Autodesk Inventor part; units mm, degrees
ref_plane "YZ Plane" through (0, 0, 0) normal (1, 0, 0) x (0, 1, 0)
ref_plane "XZ Plane" through (0, 0, 0) normal (0, 1, 0) x (-1, 0, 0)
ref_plane "XY Plane" through (0, 0, 0) normal (0, 0, 1) x (1, 0, 0)
sketch "スケッチ1" plane through (0, 0, 0) normal (0, 0, 1) x (1, 0, 0)
  line L0 (0, 0) -> (62, 0) construction
  line L1 (62, 0) -> (62, -62) construction
  line L2 (62, -62) -> (0, -62) construction
  line L3 (0, -62) -> (0, 0) construction
  line L4 (20.6, -15.3248) -> (42.6, -15.3248)
  line L5 (42.6, -15.3248) -> (42.6, -53.3248)
  line L6 (42.6, -53.3248) -> (20.6, -53.3248)
  line L7 (20.6, -53.3248) -> (20.6, -15.3248)
  circle A0 centre (26.9, -25.5248) radius 4.25
  circle A1 centre (36.3, -25.5248) radius 4.25
  dimension "d1" = 22
  dimension "d2" = 38
  dimension "d3" = 62
  dimension "d12" = 15.3248
  dimension "d16" = 20.6
  dimension "d17" = 8.5
  dimension "d18" = 8.5
  dimension "d19" = 6.3
  dimension "d25" = 10.2
  dimension "d31" = 6.3
extrude "押し出し1" add sketch "スケッチ1" along normal blind 5
sketch "スケッチ2" plane through (0, 0, 0) normal (0, 0, -1) x (-1, 0, 0)
  circle A0 centre (-36.3, -25.5248) radius 4.25
  circle A1 centre (-26.9, -25.5248) radius 4.25
  point P0 (0, 0)
extrude "押し出し2" add sketch "スケッチ2" against normal blind 12.7
equation "\"d17\" = d18"
equation "\"d31\" = d19"
properties part number "sidewindermicro2"
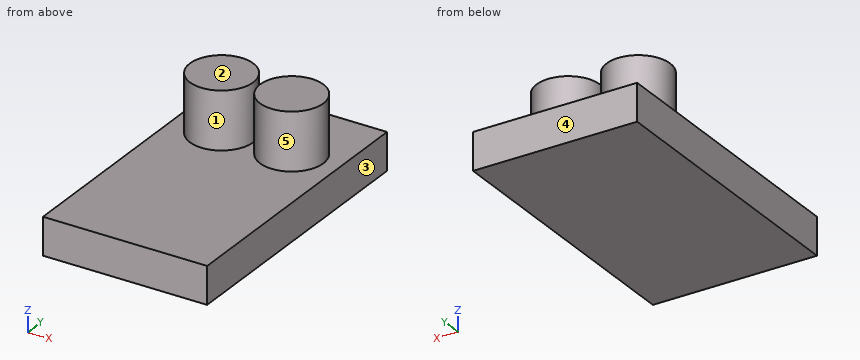
Geometry check sheet. Reference: the model listing, model coordinates, mm. Face numbers are marked on the shaded views. A direction names the side the tool comes from. Round coordinates to 2 decimals unless told otherwise and drop trailing zeros. Loops run counter-clockwise (first coordinate to the right, second up) from the corner with the lowest first, then second, coordinate; pieces in that order, holes last. Notation, with made-up numbers: M 26,25.25 L 47,25.25 A35 ccw 47,57.25 Z; hole C 35,-14.75 d7. An arc over 180 degrees is marked long. Return JSON: item names as keys, results as strings. Group by question number.
(1) Section check A-A, the plane x = 26.9. Enter the section's corners in (y, z), and give its area (3 significant figures).
(2) Go/stop test with flat-tipped pins: pin 1 (3 mm diameter, centred on x = 28.5, y = -21, fed in from -Z); pin 2 (1 mm diameter, centred on y = -22, z = 6, fed in from +X); pin 3 (5 mm diameter, centred on x = 33.5, z = 8.5, fed in from +Y). Record where each tip stops, or that it passes through.
(3) Scan lines: line 1 along Z through (x, y) = (24.5, -35.5); line 2 along X through (y, z) = (-22, 11.25); line 3 along Y through (x, z) = (35.75, 9). Record each from-to range of solid material in increasing order. Write a range as [from, to].
(4) Mould release check, pull along X, two halves, no side actions. Record for the marked faces 1, 2 and 3: pulls with the +X half, pulls with the -X half, needs draft (parallel to the pull), parting line crosses it, or undercut.
(5) Set-up check for the marked faces 4 and 5: record each of +Z, -Z, +X, -X, +Y, -Y from which the full face is reachable in a straight line by a thin tool's end or side.
(6) Section check C-C, the plane z = 8. Enter the section's corners in (x, y).
(7) Section check D-D, the plane x = 22.25. Enter the section's corners in (y, z), and give its area (3 significant figures).
(8) Section check B-B, the plane y = -22. Enter the section's corners in (x, z).
Data:
{
 "1": {"outline": "M -53.32,0 L -15.32,0 L -15.32,5 L -21.27,5 L -21.27,12.7 L -29.77,12.7 L -29.77,5 L -53.32,5 Z", "area": "255 mm²"},
 "2": {"pin 1": "z = 0", "pin 2": "x = 39.29", "pin 3": "y = -21.29"},
 "3": {"line 1": "[0, 5]", "line 2": "[24.53, 29.27], [33.93, 38.67]", "line 3": "[-29.74, -21.31]"},
 "4": {"face 1": "undercut", "face 2": "needs draft", "face 3": "pulls with the +X half"},
 "5": {"face 4": "+Z, -Z, +X, -X, +Y", "face 5": "+Z"},
 "6": {"outline": "C 26.9,-25.52 d8.5; C 36.3,-25.52 d8.5"},
 "7": {"outline": "M -53.32,0 L -15.32,0 L -15.32,5 L -53.32,5 Z", "area": "190 mm²"},
 "8": {"outline": "M 20.6,0 L 42.6,0 L 42.6,5 L 38.67,5 L 38.67,12.7 L 33.93,12.7 L 33.93,5 L 29.27,5 L 29.27,12.7 L 24.53,12.7 L 24.53,5 L 20.6,5 Z"}
}
